Source: CAD feature listing. Evaluate the final solid. Frame: model axes, mm. A direction names the side the tool comes from. Give positions to 0.01 mm unless a question says otherwise; leave off trailing zeros. Loops run counter-clockwise (first coordinate to the right, second up) from the corner with the lowest first, then second, coordinate; pieces in that order, holes last. Notation, with made-up numbers: M 11,-27.5 L 68,-27.5 A20 ccw 68,-22.5 Z; hole C 6,-31.5 d5. An arc over 180 degrees is marked long. Answer in a Markdown table with one row per item.
```python
from build123d import *

# Parameters (mm, degrees)
SKETCH_1_W               = 57
SKETCH_1_H               = 24
EXTRUDE_1_DEPTH          = 25
SKETCH_2_R               = 7.5
CUT_EXTRUDE_1_DEPTH      = 48.647668573
SKETCH_3_W               = 8
SKETCH_3_H               = 24
EXTRUDE_2_DEPTH          = 25
CUT_EXTRUDE_2_DEPTH      = 51.361473246
CUT_EXTRUDE_2_DEPTH_BACK = 51.361473246
SKETCH_5_R               = 2.5
CUT_EXTRUDE_3_DEPTH      = 43.913614482
FILLET_1_R               = 8
SKETCH_6_W               = 57
SKETCH_6_H               = 24
SKETCH_6_R               = 2.5
EXTRUDE_3_DEPTH          = 10
CUT_EXTRUDE_4_DEPTH      = 54.575183811
SKETCH_8_R               = 1.55
CUT_EXTRUDE_5_DEPTH      = 70.401572806
SKETCH_9_W               = 6
SKETCH_9_H               = 3
CUT_EXTRUDE_6_DEPTH      = 8
SKETCH_10_W              = 6
SKETCH_10_H              = 3
CUT_EXTRUDE_7_DEPTH      = 8
SKETCH_11_R              = 1.6
CUT_EXTRUDE_8_DEPTH      = 54.575183811
FILLET_2_R               = 10
FILLET_3_R               = 2
FILLET_4_R               = 2


with BuildPart() as part:
    # 草图1 → 凸台-拉伸1 (new body)
    with BuildSketch(Plane(origin=(0, 0, 0), x_dir=(1, 0, 0), z_dir=(0, 1, 0))):
        with Locations((4.200157804, -0.135814249)):
            Rectangle(SKETCH_1_W, SKETCH_1_H)
    extrude(amount=EXTRUDE_1_DEPTH)

    # 草图2 → 切除-拉伸1 (cut, through all)
    with BuildSketch(Plane.XY.offset(12.135814249)):
        with Locations((-11.799842196, 12.5)):
            Circle(SKETCH_2_R)
        with Locations((20.200157804, 12.5)):
            Circle(SKETCH_2_R)
    extrude(amount=-CUT_EXTRUDE_1_DEPTH, mode=Mode.SUBTRACT)

    # 草图3 → 凸台-拉伸2 (add)
    with BuildSketch(Plane.XZ):
        with Locations((-5.299842196, 0.135814249)):
            Rectangle(SKETCH_3_W, SKETCH_3_H)
    extrude(amount=EXTRUDE_2_DEPTH)

    # 草图4 → 切除-拉伸2 (cut, two sides: drawn at the far end of the back side and taken through both)
    with BuildSketch(Plane.ZY.offset(9.299842196).offset(-CUT_EXTRUDE_2_DEPTH_BACK)):
        with BuildLine():
            Line((-8.758359631, -19), (-8.758359631, -15))
            ThreePointArc((-8.758359631, -15), (-7.064185751, -13.30582612), (-5.370011871, -15))
            Line((-5.370011871, -15), (-5.370011871, -19))
            ThreePointArc((-5.370011871, -19), (-7.064185751, -20.69417388), (-8.758359631, -19))
        make_face()
        with BuildLine():
            Line((5.509094538, -19), (5.509094538, -15))
            ThreePointArc((5.509094538, -15), (7.235814249, -13.273280289), (8.96253396, -15))
            Line((8.96253396, -15), (8.96253396, -19))
            ThreePointArc((8.96253396, -19), (7.235814249, -20.726719711), (5.509094538, -19))
        make_face()
    extrude(amount=CUT_EXTRUDE_2_DEPTH + CUT_EXTRUDE_2_DEPTH_BACK, mode=Mode.SUBTRACT)

    # 草图5 → 切除-拉伸3 (cut, through all)
    with BuildSketch(Plane.XZ):
        with Locations(Location((4.700157804, 0.135451208, 0), (0, 0, 270))):
            Circle(SKETCH_5_R)
    extrude(amount=-CUT_EXTRUDE_3_DEPTH, mode=Mode.SUBTRACT)

    # 圆角1
    fillet_1_edges = [part.edges().sort_by_distance(p)[0] for p in [
        (-9.299842196, 0, 0.135814249),
    ]]
    fillet(fillet_1_edges, radius=FILLET_1_R)

    # 草图6 → 凸台-拉伸3 (add)
    with BuildSketch(Plane(origin=(0, 25, 0), x_dir=(1, 0, 0), z_dir=(0, 1, 0))):
        with Locations((4.200157804, -0.135814249)):
            Rectangle(SKETCH_6_W, SKETCH_6_H)
        with Locations(Location((4.700157804, -0.135451208, 0), (0, 0, 90))):
            Circle(SKETCH_6_R, mode=Mode.SUBTRACT)
    extrude(amount=EXTRUDE_3_DEPTH)

    # 草图7 → 切除-拉伸4 (cut, through all)
    with BuildSketch(Plane.XY.offset(12.135814249)):
        Polygon((-2.299842196, 25.5), (2.700157804, 25.5), (5.700157804, 25.5), (10.700157804, 25.5), (10.700157804, 16.5), (5.700157804, 16.5), (2.700157804, 16.5), (-2.299842196, 16.5), align=None)
    extrude(amount=-CUT_EXTRUDE_4_DEPTH, mode=Mode.SUBTRACT)

    # 草图8 → 切除-拉伸5 (cut, through all)
    with BuildSketch(Plane(origin=(0, 35, 0), x_dir=(1, 0, 0), z_dir=(0, 1, 0))):
        with Locations(Location((0.700157804, -7.135814249, 0), (0, 0, 270))):
            Circle(SKETCH_8_R)
        with Locations(Location((0.700157804, 6.864185751, 0), (0, 0, 270))):
            Circle(SKETCH_8_R)
    extrude(amount=-CUT_EXTRUDE_5_DEPTH, mode=Mode.SUBTRACT)

    # 草图9 → 切除-拉伸6 (cut)
    with BuildSketch(Plane.XY.offset(12.135814249)):
        with Locations((0.500157804, 30.5)):
            Rectangle(SKETCH_9_W, SKETCH_9_H)
    extrude(amount=-CUT_EXTRUDE_6_DEPTH, mode=Mode.SUBTRACT)

    # 草图10 → 切除-拉伸7 (cut)
    with BuildSketch(Plane(origin=(0, 0, -11.864185751), x_dir=(-1, 0, 0), z_dir=(0, 0, -1))):
        with Locations((-0.500157804, 30.5)):
            Rectangle(SKETCH_10_W, SKETCH_10_H)
    extrude(amount=-CUT_EXTRUDE_7_DEPTH, mode=Mode.SUBTRACT)

    # 草图11 → 切除-拉伸8 (cut, through all)
    with BuildSketch(Plane(origin=(0, 0, -11.864185751), x_dir=(-1, 0, 0), z_dir=(0, 0, -1))):
        with Locations((-28.700157804, 4)):
            Circle(SKETCH_11_R)
        with Locations((3.299842196, 4)):
            Circle(SKETCH_11_R)
    extrude(amount=-CUT_EXTRUDE_8_DEPTH, mode=Mode.SUBTRACT)

    # 圆角2
    fillet_2_edges = [part.edges().sort_by_distance(p)[0] for p in [
        (-24.299842196, 35, 0.135814249),
        (32.700157804, 35, 0.135814249),
    ]]
    fillet(fillet_2_edges, radius=FILLET_2_R)

    # 圆角3
    fillet_3_edges = [part.edges().sort_by_distance(p)[0] for p in [
        (32.700157804, 0, 0.135814249),
        (-24.299842196, 0, 0.135814249),
    ]]
    fillet(fillet_3_edges, radius=FILLET_3_R)

    # 圆角4
    fillet_4_edges = [part.edges().sort_by_distance(p)[0] for p in [
        (-9.299842196, -25, 0.135814249),
        (-1.299842196, -25, 0.135814249),
    ]]
    fillet(fillet_4_edges, radius=FILLET_4_R)


solid = part.part
```
1) Section C-C, the plane x = 6.5. Return loops of the section in (y, z), then the cut area to 3 significant figures.
Reply:
| item | result |
|---|---|
| outline | M 0,-11.86 L 16.5,-11.86 L 16.5,-1.6 L 0,-1.6 Z; M 0,1.87 L 16.5,1.87 L 16.5,12.14 L 0,12.14 Z; M 25.5,-11.86 L 35,-11.86 L 35,-1.6 L 25.5,-1.6 Z; M 25.5,1.87 L 35,1.87 L 35,12.14 L 25.5,12.14 Z |
| area | 534 mm² |
2) Set-up query: faces 1 (the flat face through (-5, -17, 5.509)), 2 (the cylindrical face through (-11.706, -2.281, 0.304)), 3 (the flat face through (-1.3, -11, 0)). Return all of +Z, -Z, +X, -X, +Y, -Y with unobstructed straight access to the full face (end or side cutting, diameter ignored); none if empty.
Reply:
| item | result |
|---|---|
| face 1 | +X, -X |
| face 2 | +Z, -Z, -X, -Y |
| face 3 | +Z, -Z, +X, -Y |
3) Pull-direction query (Y, two-part tool) for faces 4 (the flat face through (1, 32, -9)), 5 (the flat face through (-5, -25, 0)), 6 (the flat face through (4, 11, -11.864)); classes: released by +Y, released by -Y, zero draft, split by the parting line, or undercut.
Reply:
| item | result |
|---|---|
| face 4 | undercut |
| face 5 | released by -Y |
| face 6 | zero draft |
4) Material intervals for L1, parallel to X at y = 25, z = 2.75; L2, parallel to Y at x = -1, z = 1.25; L3, parallel to X at y = 31, z = 11, sorted ascending.
Reply:
| item | result |
|---|---|
| L1 | x = -24.3 to -2.3, 10.7 to 32.7 |
| L2 | y = 0 to 16.5, 25.5 to 35 |
| L3 | x = -22.3 to -2.5, 3.5 to 30.7 |
5) Pin query (flat end, axial travel): pin 1 Ø4.5 at (y, z) = (-12, 0) entering from -X; pin 2 Ø1 at (x, z) = (24.5, 7) entering from -Y; pin 3 Ø1.5 at (y, z) = (30, 7.5) entering from -X; pin 4 Ø2.5 at (x, z) = (0.7, 7.14) entering from +Y. Return the tip coordinate at first contact, or that it passes through.
Reply:
| item | result |
|---|---|
| pin 1 | stops at x = -9.3 |
| pin 2 | stops at y = 0 |
| pin 3 | stops at x = -23.35 |
| pin 4 | passes through |
6) Section B-B, the plane x = 21. Return loops of the section in (y, z), then the cut area to 3 significant figures.
Reply:
| item | result |
|---|---|
| outline | M 0,-11.86 L 5.04,-11.86 L 5.04,12.14 L 0,12.14 Z; M 19.96,-11.86 L 35,-11.86 L 35,12.14 L 19.96,12.14 Z |
| area | 482 mm² |
7) Section D-D, the plane y = 4. Return loops of the section in (x, z).
Reply:
| item | result |
|---|---|
| outline | M -24.3,-11.86 L -4.9,-11.86 L -4.9,12.14 L -24.3,12.14 Z; M -1.7,-11.86 L 27.1,-11.86 L 27.1,12.14 L -1.7,12.14 Z; M 30.3,-11.86 L 32.7,-11.86 L 32.7,12.14 L 30.3,12.14 Z; hole C 0.7,-6.86 d3.1; hole C 0.7,7.14 d3.1; hole C 4.7,0.14 d5 |
8) Section A-A, the plane y = 12.5. Return loops of the section in (x, z), then the cut area to 3 significant figures.
Reply:
| item | result |
|---|---|
| outline | M -24.3,-11.86 L -19.3,-11.86 L -19.3,12.14 L -24.3,12.14 Z; M -4.3,-11.86 L 12.7,-11.86 L 12.7,12.14 L -4.3,12.14 Z; M 27.7,-11.86 L 32.7,-11.86 L 32.7,12.14 L 27.7,12.14 Z; hole C 0.7,-6.86 d3.1; hole C 0.7,7.14 d3.1; hole C 4.7,0.14 d5 |
| area | 613 mm² |
